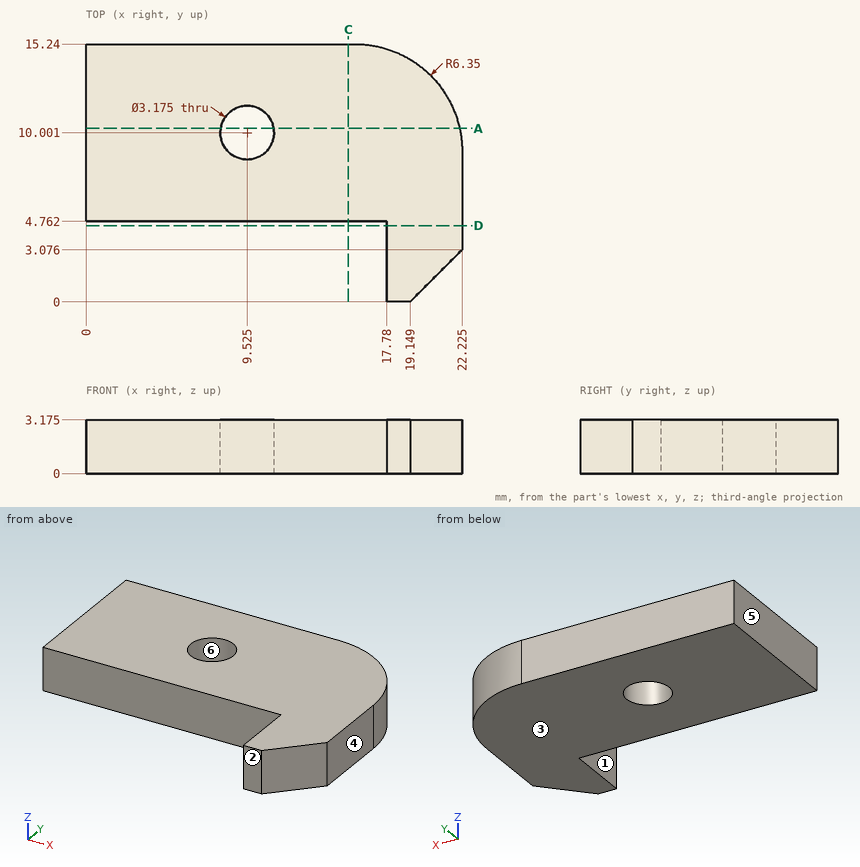
Print and shaded views of the part. All mm, measured from the part's lowest x, y and z. A direction names the side the tool comes from. Round coordinates to 2 decimals unless told otherwise and drop trailing zeros. Write each loop counter-clockwise with the first axis right and the second up, starting at its lowest first coordinate (ties: lowest second). Pieces come first, ordered by that corner, then holes. Notation, with made-up numbers: M 47.25,71 L 59.25,71 A21 cw 59.25,89 Z; hole C 54.5,-1 d2. An arc over 180 degrees is marked long. Use a Markdown table: item, result. Add a question column.
1. Slice it at C-C on x = 15.5. Give the cut face in (y, z) (1 decimal).
2. Drill centre lines: probe 1 along Y at (x, z) = (9.5, 1.45); probe 2 along Y at (x, z) = (1.75, 1.95); probe 3 along X at (y, z) = (10, 1.1). Where is each one in solid material? Low to high.
3. Slice it at D-D on y = 4.5. Give the cut face in (x, z) (1 decimal).
4. 3-axis set-ups, long thin cutter, end or side, ignore diameter. For the marked faces 1 and 2: which of +Z, -Z, +X, -X, +Y, -Y reach the whole face in a straight line?
5. Slice it at A-A on y = 10.25. Give the cut face in (x, z) (1 decimal).
6. Pull direction X, two halves, no side cores. Call the marked faces 3, 4, 5 and 6: released by +X, released by -X, zero draft, split by the parting line, or undercut.
7. Flat gauge pin, fed straight in: P1, Ø1, axis at y = 3, z = 2, coming from the -X side. Where does the tip first touch, or does it go through?
Reply:
| question | item | result |
|---|---|---|
| 1 | outline | M 4.8,0 L 15.2,0 L 15.2,3.2 L 4.8,3.2 Z |
| 2 | probe 1 | y = 4.76 to 8.41, 11.59 to 15.24 |
| 2 | probe 2 | y = 4.76 to 15.24 |
| 2 | probe 3 | x = 0 to 7.94, 11.11 to 22.13 |
| 3 | outline | M 17.8,0 L 22.2,0 L 22.2,3.2 L 17.8,3.2 Z |
| 4 | face 1 | +Z, -Z, -X, -Y |
| 4 | face 2 | +Z, -Z, +X, -X, -Y |
| 5 | outline | M 0,0 L 8,0 L 8,3.2 L 0,3.2 Z; M 11.1,0 L 22.1,0 L 22.1,3.2 L 11.1,3.2 Z |
| 6 | face 3 | zero draft |
| 6 | face 4 | released by +X |
| 6 | face 5 | released by -X |
| 6 | face 6 | undercut |
| 7 | P1 | stops at x = 17.78 |
